```python
from build123d import *

# Parameters (mm, degrees)
F1_DEPTH = 900
F2_W     = 900
F2_H     = 100
F3_DEPTH = 900
F5_DEPTH = 70
F7_W     = 40
F7_H     = 40
F8_DEPTH = 306


with BuildPart() as f1:
    # F0 (on Front) → F1 (new body)
    with BuildSketch(Plane.XZ):
        with BuildLine():
            ThreePointArc((0, 20), (5.8578643763, 5.8578643763), (20, 0))
            Line((20, 0), (1130, 0))
            ThreePointArc((1130, 0), (1144.1421356237, 5.8578643763), (1150, 20))
            Line((1150, 20), (1150, 80))
            ThreePointArc((1150, 80), (1144.1421356237, 94.1421356237), (1130, 100))
            Line((1130, 100), (20, 100))
            ThreePointArc((20, 100), (5.8578643763, 94.1421356237), (0, 80))
            Line((0, 80), (0, 20))
        make_face()
    extrude(amount=-F1_DEPTH)

    # F2 (on Front) → F3 (join, through all)
    with BuildSketch(Plane.XZ):
        with Locations((450, -50)):
            Rectangle(F2_W, F2_H)
    extrude(amount=-F3_DEPTH)

    # F4 (on face) → F5 (join)
    with BuildSketch(Plane.XZ):
        with BuildLine():
            ThreePointArc((1137.4171255462, 35.8593240664), (1139.3489836073, 42.8126855449), (1140, 50))
            ThreePointArc((1140, 50), (1113.0987167635, 87.7944919155), (1068.5788190425, 74.752967241))
            ThreePointArc((1068.5788190425, 74.752967241), (1080.3234477683, 15.1742438377), (1137.4171255462, 35.8593240664))
        make_face()
        with BuildLine():
            ThreePointArc((1137.4171255462, 35.8593240664), (1080.3234477683, 15.1742438377), (1068.5788190425, 74.752967241))
            Line((1068.5788190425, 74.752967241), (928.0852857046, -103.5881864231))
            ThreePointArc((928.0852857046, -103.5881864231), (1011.5600939315, -79.1353276584), (1062, -150))
            ThreePointArc((1062, -150), (1060.7793442636, -163.4762146032), (1057.1571103991, -176.5137673755))
            Line((1057.1571103991, -176.5137673755), (1137.4171255462, 35.8593240664))
        make_face()
        with BuildLine():
            ThreePointArc((1062, -150), (1011.5600939315, -79.1353276584), (928.0852857046, -103.5881864231))
            ThreePointArc((928.0852857046, -103.5881864231), (950.1064645656, -215.2982928043), (1057.1571103991, -176.5137673755))
            ThreePointArc((1057.1571103991, -176.5137673755), (1060.7793442636, -163.4762146032), (1062, -150))
        make_face()
    extrude(amount=F5_DEPTH)

    # F7 (on offset) → F8 (join, through all)
    with BuildSketch(Plane(origin=(0, 0, -406), x_dir=(1, 0, 0), z_dir=(0, 0, -1))):
        with Locations((335, -20.0000000002)):
            Rectangle(F7_W, F7_H)
        with Locations((335, -880.0000000002)):
            Rectangle(F7_W, F7_H)
        with Locations((815, -20.0000000002)):
            Rectangle(F7_W, F7_H)
        with Locations((815, -880.0000000002)):
            Rectangle(F7_W, F7_H)
    extrude(amount=-F8_DEPTH)


solid = f1.part
```
Check sheet for the modelled part. Datum: model origin and axes. Units: mm. A direction names the side the tool comes from. Round coordinates to 2 decimals unless told otherwise and drop trailing zeros. Order: outer loops, then holes, each group sorted by start corner. A loop starts at its lowest first (then second) coordinate and runs counter-clockwise, first axis right, second up. Notation, with made-up numbers: (4, 52) -> (62, 52) arc R17 cw to (62, 73) -> close; hole circle Ø8 at (88.5, 15.25). An arc over 180 degrees is marked (long way). One line per item, written item: value. Start each with the question number.
Q1. Cross-section at D-D (y = 291). Record the boundary of the cut face in (x, z).
Q2. Mould release check, pull along Y, two halves, no side actions. Record for faces 1 (the face through (815, 860, -255)), 2 (the face through (1096.725, -34.51, -71.814)): pulls with the +Y half, pulls with the -Y half, needs draft (parallel to the pull), parting line crosses it, or undercut.
Q3. Cross-section at A-A (z = -366). Record the boundary of the cut face in (x, y), and give its area (3 significant figures).
Q4. Cross-section at B-B (z = -26.5). Record the boundary of the cut face in (x, y), and give its area (3 significant figures).
Q5. Thickness scan on line 1 (X direction, y = 3.5, z = -285); line 2 (Y direction, x = 378, z = 30.5); line 3 (Z direction, x = 326, y = 386.5). Record the ranges inside material, lowest first.
Q6. Gauge pin test, flat ends, axial feed: pin 1 Ø12 at (y, z) = (878, -191) entering from +X; pin 2 Ø10 at (x, y) = (8, 493) entering from +Z (3 decimals); pin 3 Ø12 at (x, z) = (323.5, -189) entering from -Y. Record the tip position at first contact, or that the pin passes through.
Q7. Set-up check for faces 3 (the face through (315, 20, -255)), 4 (the face through (900, 444, -51)), 5 (the face through (795, 880, -255)), 6 (the face through (335, 860, -255)): record each of +Z, -Z, +X, -X, +Y, -Y from which the full face is reachable in a straight line by a thin tool's end or side.
Q8. Cross-section at C-C (x = 987). Record the boundary of the cut face in (y, z).
Completed:
1. outline: (0, -100) -> (900, -100) -> (900, 0) -> (1130, 0) arc R20 ccw to (1150, 20) -> (1150, 80) arc R20 ccw to (1130, 100) -> (20, 100) arc R20 ccw to (0, 80) -> (0, 20) arc R20 ccw to (20, 0) -> (0, 0) -> close
2. face 1: undercut
2. face 2: needs draft
3. outline: (315, 0) -> (355, 0) -> (355, 40) -> (315, 40) -> close; (315, 860) -> (355, 860) -> (355, 900) -> (315, 900) -> close; (795, 0) -> (835, 0) -> (835, 40) -> (795, 40) -> close; (795, 860) -> (835, 860) -> (835, 900) -> (795, 900) -> close
3. area: 6,400 mm²
4. outline: (0, 0) -> (900, 0) -> (900, 900) -> (0, 900) -> close; (988.81, -70) -> (1113.85, -70) -> (1113.85, 0) -> (988.81, 0) -> close
4. area: 819,000 mm²
5. line 1: x = 315 to 355, 795 to 835
5. line 2: y = 0 to 900
5. line 3: z = -100 to 100
6. pin 1: stops at x = 835
6. pin 2: stops at z = 98.735
6. pin 3: stops at y = 0
7. face 3: -Z, -X, +Y, -Y
7. face 4: -Z, +X, +Y, -Y
7. face 5: -Z, +Y, -Y
7. face 6: -Z, +X, -X
8. outline: (-70, -225) -> (0, -225) -> (0, -28.8) -> (-70, -28.8) -> close; (0, 0) -> (900, 0) -> (900, 100) -> (0, 100) -> close
